Source: CAD feature listing. Evaluate the final solid. Frame: model axes, mm. A direction names the side the tool comes from. Give positions to 0.01 mm unless a question says otherwise; leave off trailing zeros. Loops run counter-clockwise (first coordinate to the right, second up) from the corner with the lowest first, then second, coordinate; pieces in that order, holes last.
```python
from build123d import *

# Parameters (mm, degrees)
BOSS_EXTRUDE1_DEPTH = 3
SKETCH2_W           = 130
SKETCH2_H           = 1.5
BOSS_EXTRUDE2_DEPTH = 3
SKETCH3_W           = 1.5
SKETCH3_H           = 11.641666667
SKETCH3_H_2         = 11.641666666
BOSS_EXTRUDE3_DEPTH = 3
SKETCH4_R           = 2
CUT_EXTRUDE1_DEPTH  = 97.213304693


with BuildPart() as part:
    # Sketch1 → Boss-Extrude1 (new body)
    with BuildSketch(Plane(origin=(0, 0, 0), x_dir=(1, 0, 0), z_dir=(0, 1, 0))):
        Polygon((65, 38.88), (68, 38.88), (68, 12.76), (65, 12.76), (65, -13.06), (68, -13.06), (68, -39.18), (65, -39.18), (65, -65), (39.18, -65), (39.18, -68), (13.06, -68), (13.06, -65), (-12.76, -65), (-12.76, -68), (-38.88, -68), (-38.88, -65), (-64.7, -65), (-68, -65), (-68, -38.88), (-65, -38.88), (-65, -13.06), (-68, -13.06), (-68, 13.06), (-65, 13.06), (-65, 38.88), (-68, 38.88), (-68, 65), (-65, 65), (-65, 68), (-38.88, 68), (-38.88, 65), (-13.06, 65), (-13.06, 68), (13.06, 68), (13.06, 65), (38.88, 65), (38.88, 68), (65, 68), (65, 64.7), align=None)
        with BuildLine():
            Line((11.149299305, -38.675), (-11.149299305, -38.675))
            ThreePointArc((-11.149299305, -38.675), (-28.461047943, -28.461047943), (-38.675, -11.149299305))
            Line((-38.675, -11.149299305), (-38.675, 11.149299305))
            ThreePointArc((-38.675, 11.149299305), (-28.461047943, 28.461047943), (-11.149299305, 38.675))
            Line((-11.149299305, 38.675), (11.149299305, 38.675))
            ThreePointArc((11.149299305, 38.675), (28.461047943, 28.461047943), (38.675, 11.149299305))
            Line((38.675, 11.149299305), (38.675, -11.149299305))
            ThreePointArc((38.675, -11.149299305), (28.461047943, -28.461047943), (11.149299305, -38.675))
        make_face(mode=Mode.SUBTRACT)
    extrude(amount=BOSS_EXTRUDE1_DEPTH)

    # Sketch2 → Boss-Extrude2 (add, through all)
    with BuildSketch(Plane(origin=(0, 3, 0), x_dir=(1, 0, 0), z_dir=(0, 1, 0))):
        with Locations((0, 39.425)):
            Rectangle(SKETCH2_W, SKETCH2_H)
        with Locations((0, 26.283333333)):
            Rectangle(SKETCH2_W, SKETCH2_H)
        with Locations((0, 13.141666667)):
            Rectangle(SKETCH2_W, SKETCH2_H)
        Rectangle(SKETCH2_W, SKETCH2_H)
        with Locations((0, -13.141666667)):
            Rectangle(SKETCH2_W, SKETCH2_H)
        with Locations((0, -26.283333333)):
            Rectangle(SKETCH2_W, SKETCH2_H)
        with Locations((0, -39.425)):
            Rectangle(SKETCH2_W, SKETCH2_H)
    extrude(amount=-BOSS_EXTRUDE2_DEPTH)

    # Sketch3 → Boss-Extrude3 (add, through all)
    with BuildSketch(Plane(origin=(0, 3, 0), x_dir=(1, 0, 0), z_dir=(0, 1, 0))):
        with Locations((-19.7125, -6.570833334)):
            Rectangle(SKETCH3_W, SKETCH3_H)
        with Locations((-19.7125, 6.570833334)):
            Rectangle(SKETCH3_W, SKETCH3_H)
        with Locations((-19.7125, -19.7125)):
            Rectangle(SKETCH3_W, SKETCH3_H_2)
        with Locations((0, -6.570833334)):
            Rectangle(SKETCH3_W, SKETCH3_H)
        with Locations((-19.7125, 19.7125)):
            Rectangle(SKETCH3_W, SKETCH3_H_2)
        with Locations((0, 6.570833334)):
            Rectangle(SKETCH3_W, SKETCH3_H)
        with BuildLine():
            Line((-18.9625, -27.033333333), (-20.4625, -27.033333333))
            Line((-20.4625, -27.033333333), (-20.4625, -34.66047596))
            ThreePointArc((-20.4625, -34.66047596), (-19.717004208, -35.089916573), (-18.9625, -35.503325108))
            Line((-18.9625, -35.503325108), (-18.9625, -27.033333333))
        make_face()
        with Locations((0, -19.7125)):
            Rectangle(SKETCH3_W, SKETCH3_H_2)
        with Locations((19.7125, -6.570833334)):
            Rectangle(SKETCH3_W, SKETCH3_H)
        with BuildLine():
            Line((-20.4625, 34.66047596), (-20.4625, 27.033333333))
            Line((-20.4625, 27.033333333), (-18.9625, 27.033333333))
            Line((-18.9625, 27.033333333), (-18.9625, 35.503325108))
            ThreePointArc((-18.9625, 35.503325108), (-19.717004208, 35.089916573), (-20.4625, 34.66047596))
        make_face()
        with Locations((0, 19.7125)):
            Rectangle(SKETCH3_W, SKETCH3_H_2)
        with Locations((19.7125, 6.570833334)):
            Rectangle(SKETCH3_W, SKETCH3_H)
        with Locations((0, -32.854166667)):
            Rectangle(SKETCH3_W, SKETCH3_H)
        with Locations((19.7125, -19.7125)):
            Rectangle(SKETCH3_W, SKETCH3_H_2)
        with Locations((0, 32.854166667)):
            Rectangle(SKETCH3_W, SKETCH3_H)
        with Locations((19.7125, 19.7125)):
            Rectangle(SKETCH3_W, SKETCH3_H_2)
        with BuildLine():
            Line((20.4625, -27.033333333), (18.9625, -27.033333333))
            Line((18.9625, -27.033333333), (18.9625, -35.503325108))
            ThreePointArc((18.9625, -35.503325108), (19.717004208, -35.089916573), (20.4625, -34.66047596))
            Line((20.4625, -34.66047596), (20.4625, -27.033333333))
        make_face()
        with BuildLine():
            Line((18.9625, 35.503325108), (18.9625, 27.033333333))
            Line((18.9625, 27.033333333), (20.4625, 27.033333333))
            Line((20.4625, 27.033333333), (20.4625, 34.66047596))
            ThreePointArc((20.4625, 34.66047596), (19.717004208, 35.089916573), (18.9625, 35.503325108))
        make_face()
    extrude(amount=-BOSS_EXTRUDE3_DEPTH)

    # Sketch4 → Cut-Extrude1 (cut, through all)
    with BuildSketch(Plane(origin=(0, 3, 0), x_dir=(1, 0, 0), z_dir=(0, 1, 0))):
        with Locations(Location((-35.75, 35.75, 0), (0, 0, 270))):
            Circle(SKETCH4_R)
        with Locations(Location((35.75, 35.75, 0), (0, 0, 270))):
            Circle(SKETCH4_R)
        with Locations(Location((35.75, -35.75, 0), (0, 0, 270))):
            Circle(SKETCH4_R)
        with Locations(Location((-35.75, -35.75, 0), (0, 0, 270))):
            Circle(SKETCH4_R)
    extrude(amount=-CUT_EXTRUDE1_DEPTH, mode=Mode.SUBTRACT)


solid = part.part
```
(1) Section A-A, the plane z = 8.5. Count the separate pieces of the cut face and the enclosed holes in it, then the cut area to 3 significant figures.
A:
separate pieces: 5
enclosed holes: 0
area: 180 mm2
(2) Section D-D, the plane z = 29. Return the cut outline in (x, y), then the cut area to 3 significant figures.
A:
outline: (-65, 0) - (-27.91, 0) - (-27.91, 3) - (-65, 3) - close; (-20.46, 0) - (-18.96, 0) - (-18.96, 3) - (-20.46, 3) - close; (-0.75, 0) - (0.75, 0) - (0.75, 3) - (-0.75, 3) - close; (18.96, 0) - (20.46, 0) - (20.46, 3) - (18.96, 3) - close; (27.91, 0) - (68, 0) - (68, 3) - (27.91, 3) - close
area: 245 mm2
(3) Reachability of faces 4 (the flat face through (-38.88, 1, -67)), 5 (the flat face through (67, 1, 39.18)), 6 (the flat face through (18.962, 2, 7)), 7 (the flat face through (13.06, 1, 67)) from +Z, -Z, +X, -X, +Y, -Y: full face, straight path, thin tool, end or side. Return the list, or none.
A:
face 4: -Z, +Y, -Y
face 5: +Z, +X, +Y, -Y
face 6: +Y, -Y
face 7: +Z, +Y, -Y
(4) Ray query, line 1 along X through (y, z) = (2.7, -20.5); line 2 along X through (y, z) = (2.45, -29.5); line 3 along X through (y, z) = (1.1, 41.5). Return the intervals inside material, ascending.
A:
line 1: x = -65 to -34.64, -20.46 to -18.96, -0.75 to 0.75, 18.96 to 20.46, 34.64 to 68
line 2: x = -65 to -27.38, -20.46 to -18.96, -0.75 to 0.75, 18.96 to 20.46, 27.38 to 68
line 3: x = -68 to 65
(5) First-contact query: pin 1 (1.5 mm diameter, centred on y = 2, z = -33.5, fed in from -X); pin 2 (0.9 mm diameter, centred on x = 48, y = 1, fed in from +Z); pin 3 (1.5 mm diameter, centred on y = 1.5, z = 66.5, fed in from -X). Flat tips, straight axial feed; report the tip coordinate or a pass-through.
A:
pin 1: stops at x = -65
pin 2: stops at z = 65
pin 3: stops at x = -38.88
(6) Mould query, pull axis X, two halves, no side actions, for faces 1 (the flat face through (-67, 1, -65)), 2 (the flat face through (-25, 2, -27.033)), 3 (the flat face through (18.962, 2, -20)). Classes: pulls with the +X half, pulls with the -X half, needs draft (parallel to the pull), parting line crosses it, or undercut.
A:
face 1: needs draft
face 2: undercut
face 3: undercut
(7) Section B-B, the plane x = -35.75. Return the cut outline in (y, z).
A:
outline: (0, -65) - (3, -65) - (3, -37.75) - (0, -37.75) - close; (0, -33.75) - (3, -33.75) - (3, -18.49) - (0, -18.49) - close; (0, -13.89) - (3, -13.89) - (3, -12.39) - (0, -12.39) - close; (0, -0.75) - (3, -0.75) - (3, 0.75) - (0, 0.75) - close; (0, 12.39) - (3, 12.39) - (3, 13.89) - (0, 13.89) - close; (0, 18.49) - (3, 18.49) - (3, 33.75) - (0, 33.75) - close; (0, 37.75) - (3, 37.75) - (3, 68) - (0, 68) - close
